from build123d import *

# Parameters (mm, degrees)
F1_DEPTH     = 19.05
F2_R         = 15.059033574
F3_DEPTH     = 3.81
F6_DEPTH     = 25.4
F8_DEPTH     = 98.4172728563
F4_R         = 4.2206847971
F9_DEPTH     = 25.4
F10_SIZE     = 3.80999
F11_R        = 12.7
F12_R        = 12.7
F13_R        = 7.62
F14_R        = 5.08
F15_R        = 7.62
F16_R        = 7.62
F17_R        = 5.08
F18_R        = 7.62
F19_R        = 5.08
F20_T1_DEPTH = 19.05
F21_R        = 2.54
F22_R        = 15.24


# Not quite as in the source:
# - a fillet or chamfer that OpenCascade refuses, or shapes differently, is made with other operations: its cross-section is extruded or revolved along the edge and cut away or added
# - a fillet or chamfer is up to 0.001 mm smaller than in the source, because OpenCascade refuses the exact size


with BuildPart() as f1:
    # F0 (on Top) → F1 (new body)
    with BuildSketch(Plane.XY):
        Polygon((57.15, 90.8419879414), (0, 90.8419879414), (-57.15, 90.8419879414), (-47.625, -86.9580120586), (0, -86.9580120586), (47.625, -86.9580120586), align=None)
        with BuildLine():
            Line((-39.8510134111, -64.9218410254), (-19.0060128585, -64.9218410254))
            ThreePointArc((-19.0060128585, -64.9218410254), (-15.7100075961, -71.1253052436), (-10.4695623741, -75.8033767343))
            Line((-10.4695623741, -75.8033767343), (-10.4695623741, -78.8165818754))
            Line((-10.4695623741, -78.8165818754), (-40.5953745281, -78.8165818754))
            Line((-40.5953745281, -78.8165818754), (-39.8510134111, -64.9218410254))
        make_face(mode=Mode.SUBTRACT)
        with BuildLine():
            Line((-42.0940332115, -10.5141438544), (-10.4695623741, -10.5141438544))
            Line((-10.4695623741, -10.5141438544), (-10.4695623741, -41.7985618114))
            ThreePointArc((-10.4695623741, -41.7985618114), (-15.6132317705, -46.3542592872), (-18.9080441845, -52.3838467943))
            Line((-18.9080441845, -52.3838467943), (-39.8510134111, -52.3838467943))
            Line((-39.8510134111, -52.3838467943), (-42.0940332115, -10.5141438544))
        make_face(mode=Mode.SUBTRACT)
        with BuildLine():
            Line((19.0060128585, -64.9218410254), (39.8510134111, -64.9218410254))
            Line((39.8510134111, -64.9218410254), (40.5953745281, -78.8165818754))
            Line((40.5953745281, -78.8165818754), (10.4695623741, -78.8165818754))
            Line((10.4695623741, -78.8165818754), (10.4695623741, -75.8033767343))
            ThreePointArc((10.4695623741, -75.8033767343), (15.7100075961, -71.1253052436), (19.0060128585, -64.9218410254))
        make_face(mode=Mode.SUBTRACT)
        with BuildLine():
            Line((10.4695623741, -10.5141438544), (42.0940332115, -10.5141438544))
            Line((42.0940332115, -10.5141438544), (39.8510134111, -52.3838467943))
            Line((39.8510134111, -52.3838467943), (18.9080441845, -52.3838467943))
            ThreePointArc((18.9080441845, -52.3838467943), (15.6132317705, -46.3542592872), (10.4695623741, -41.7985618114))
            Line((10.4695623741, -41.7985618114), (10.4695623741, -10.5141438544))
        make_face(mode=Mode.SUBTRACT)
        Polygon((-10.4695623741, 71.0973963141), (-10.4695623741, 4.7880196944), (-42.0940332115, 4.7880196944), (-45.4945191741, 71.0973963141), align=None, mode=Mode.SUBTRACT)
        Polygon((10.4695623741, 4.7880196944), (10.4695623741, 71.0973963141), (45.4945191741, 71.0973963141), (42.0940332115, 4.7880196944), align=None, mode=Mode.SUBTRACT)
    extrude(amount=F1_DEPTH)

    # F2 (on face) → F3 (join)
    with BuildSketch(Plane.XY.offset(19.05)):
        with Locations((0, -58.8009692729)):
            Circle(F2_R)
    extrude(amount=F3_DEPTH)

    # F5 (on face) → F6 (join)
    with BuildSketch(Plane.XY.offset(19.05)):
        Polygon((15.6109640375, 85.8776420355), (0, 85.8776420355), (-15.6109640375, 85.8776420355), (-15.6109640375, 76.2544423342), (0, 76.2544423342), (15.6109640375, 76.2544423342), align=None)
        Polygon((-15.6109640375, -7.5742849149), (0, -7.5742849149), (15.6109640375, -7.5742849149), (15.6109640375, 2.0489108283), (0, 2.0489108283), (-15.6109640375, 2.0489108283), align=None)
    extrude(amount=F6_DEPTH)

    # F7 (on face) → F8 (cut, through all)
    with BuildSketch(Plane.XZ.offset(7.5742849149)):
        Polygon((3.81, 35.5143319389), (0, 35.5143319389), (-3.81, 35.5143319389), (-3.81, 27.8943319389), (0, 27.8943319389), (3.81, 27.8943319389), align=None)
    extrude(amount=-F8_DEPTH, mode=Mode.SUBTRACT)

    # F4 (on face) → F9 (join)
    with BuildSketch(Plane.XY.offset(22.86)):
        with Locations((0, -58.8009692729)):
            Circle(F4_R)
    extrude(amount=F9_DEPTH)

    # F10 (size 3.81 in the source; OpenCascade refuses exactly that, so slightly less here)
    f10_edges = [f1.edges().sort_by_distance(p)[0] for p in [
        (-15.059034, -58.800969, 22.86),
    ]]
    chamfer(f10_edges, length=F10_SIZE)

    # F11
    f11_edges = [f1.edges().sort_by_distance(p)[0] for p in [
        (15.610964, -2.762687, 44.45),
        (-15.610964, -2.762687, 44.45),
    ]]
    fillet(f11_edges, radius=F11_R)

    # F12
    f12_edges = [f1.edges().sort_by_distance(p)[0] for p in [
        (15.610964, 81.066042, 44.45),
        (-15.610964, 81.066042, 44.45),
    ]]
    fillet(f12_edges, radius=F12_R)

    # F13
    f13_edges = [f1.edges().sort_by_distance(p)[0] for p in [
        (-45.494519, 71.097396, 9.525),
    ]]
    fillet(f13_edges, radius=F13_R)

    # F14
    f14_edges = [f1.edges().sort_by_distance(p)[0] for p in [
        (-42.094033, -10.514144, 9.525),
    ]]
    fillet(f14_edges, radius=F14_R)

    # F15
    f15_edges = [f1.edges().sort_by_distance(p)[0] for p in [
        (-10.469562, 71.097396, 9.525),
        (45.494519, 71.097396, 9.525),
    ]]
    fillet(f15_edges, radius=F15_R)

    # F16
    f16_edges = [f1.edges().sort_by_distance(p)[0] for p in [
        (-42.094033, 4.78802, 9.525),
        (10.469562, 4.78802, 9.525),
    ]]
    fillet(f16_edges, radius=F16_R)

    # F17
    f17_edges = [f1.edges().sort_by_distance(p)[0] for p in [
        (-10.469562, 4.78802, 9.525),
        (42.094033, 4.78802, 9.525),
    ]]
    fillet(f17_edges, radius=F17_R)

    # F18
    f18_edges = [f1.edges().sort_by_distance(p)[0] for p in [
        (10.469562, 71.097396, 9.525),
    ]]
    fillet(f18_edges, radius=F18_R)

    # F19
    f19_edges = [f1.edges().sort_by_distance(p)[0] for p in [
        (-10.469562, -10.514144, 9.525),
        (42.094033, -10.514144, 9.525),
        (10.469562, -10.514144, 9.525),
        (-39.851013, -52.383847, 9.525),
        (39.851013, -52.383847, 9.525),
    ]]
    fillet(f19_edges, radius=F19_R)

    # F20: fillet of radius 5.08 on 6 edges, made by hand

    # F20_s2 → F20_t1 (join)
    with BuildSketch(Plane.XY):
        with BuildLine():
            ThreePointArc((40.3086734646, -73.4648286909), (38.9228773885, -77.2312845683), (35.2359473527, -78.8165818754))
            Line((35.2359473527, -78.8165818754), (40.5953745281, -78.8165818754))
            Line((40.5953745281, -78.8165818754), (40.3086734646, -73.4648286909))
        make_face()
        with BuildLine():
            ThreePointArc((-15.1101182687, -78.8165818754), (-12.3436148694, -77.9971990774), (-10.4695623741, -75.8033767343))
            Line((-10.4695623741, -75.8033767343), (-10.4695623741, -78.8165818754))
            Line((-10.4695623741, -78.8165818754), (-15.1101182687, -78.8165818754))
        make_face()
        with BuildLine():
            ThreePointArc((-40.3086734646, -73.4648286909), (-38.9228773885, -77.2312845683), (-35.2359473527, -78.8165818754))
            Line((-35.2359473527, -78.8165818754), (-40.5953745281, -78.8165818754))
            Line((-40.5953745281, -78.8165818754), (-40.3086734646, -73.4648286909))
        make_face()
        with BuildLine():
            ThreePointArc((10.4695623741, -75.8033767343), (12.3436148694, -77.9971990774), (15.1101182687, -78.8165818754))
            Line((15.1101182687, -78.8165818754), (10.4695623741, -78.8165818754))
            Line((10.4695623741, -78.8165818754), (10.4695623741, -75.8033767343))
        make_face()
        with BuildLine():
            ThreePointArc((35.03587195, -64.9218410254), (38.5305746428, -66.3149109896), (40.1085980619, -69.7300878408))
            Line((40.1085980619, -69.7300878408), (39.8510134111, -64.9218410254))
            Line((39.8510134111, -64.9218410254), (35.03587195, -64.9218410254))
        make_face()
        with BuildLine():
            ThreePointArc((-35.03587195, -64.9218410254), (-38.5305746428, -66.3149109896), (-40.1085980619, -69.7300878408))
            Line((-40.1085980619, -69.7300878408), (-39.8510134111, -64.9218410254))
            Line((-39.8510134111, -64.9218410254), (-35.03587195, -64.9218410254))
        make_face()
    extrude(amount=F20_T1_DEPTH)

    # F21
    f21_edges = [f1.edges().sort_by_distance(p)[0] for p in [
        (10.469562, -75.803377, 9.525),
        (-10.469562, -75.803377, 9.525),
    ]]
    fillet(f21_edges, radius=F21_R)

    # F22
    f22_edges = [f1.edges().sort_by_distance(p)[0] for p in [
        (-47.625, -86.958012, 9.525),
        (-57.15, 90.841988, 9.525),
        (57.15, 90.841988, 9.525),
        (47.625, -86.958012, 9.525),
    ]]
    fillet(f22_edges, radius=F22_R)


solid = f1.part
The model under review builds one solid part; all positions refer to its coordinate system, in mm. A direction names the side the tool comes from. Give positions to 0.01 mm unless a question says otherwise; leave off trailing zeros. Write each loop counter-clockwise with the first axis right and the second up, starting at its lowest first coordinate (ties: lowest second). Pieces come first, ordered by that corner, then holes.
1. Wall thickness on L1, parallel to Y at x = 28.5, z = 15; L2, parallel to Y at x = -38.5, z = 10; L3, parallel to Z at x = -1.5, y = 0.5: over which ranges is each line inside the solid? List them lowest first.
2. For P1, Ø3, axis at x = 12.5, z = 41, coming from the +Y side; P2, Ø4, axis at x = 28, y = 69.5, coming from the +Z side; P3, Ø4, axis at y = 58.5, z = 6.5, coming from the -X side; P4, Ø8, axis at x = 35.5, z = 6.5, coming from the -Y side, all flat-tipped, find the tip position at first contact; note any pin that passes through.
3. Draft analysis for pull direction Z (two halves, no side actions). For faces 1 (the flat face through (5, -59, 22.86)), 2 (the flat face through (0, -3, 35.514)), 3 (the flat face through (-28, 71.097, 9)), state which applies: +Z half, -Z half, draft (parallel to the pull), parting line (faces both ways), or undercut.
4. Add section C-C, the plane x = 28.5. Write out the cut boundary in (y, z), plus the area to 3 significant figures.
5. Add section A-A, the plane x = 0. Count the separate pieces of the cut face and the enclosed holes in it, plus the area to 3 significant figures.
6. Add section B-B, the plane y = 60. Write out the cut boundary in (x, z).
7. Tool access review of faces 4 (the cylindrical face through (16.48, -70.075, 9.392)), 5 (the flat face through (0, -3, 27.894)), 6 (the flat face through (1, 90.842, 9)): name each direction out of +Z, -Z, +X, -X, +Y, -Y from which nothing blocks a thin tool from reaching the whole face with its end or side.
Worked answers:
1. L1: y = -86.96 to -78.82, -64.92 to -52.38, -10.51 to 4.79, 71.1 to 90.84
1. L2: y = -86 to -77.63, -66.29 to -51.02, -10.83 to 5.72, 71.03 to 90.84
1. L3: z = 0 to 27.89, 35.51 to 44.45
2. P1: stops at y = 85.88
2. P2: stops at z = 19.05
2. P3: stops at x = -55.52
2. P4: stops at y = -86.96
3. face 1: +Z half
3. face 2: undercut
3. face 3: draft
4. outline: (-86.96, 0) - (-78.82, 0) - (-78.82, 19.05) - (-86.96, 19.05) - close; (-64.92, 0) - (-52.38, 0) - (-52.38, 19.05) - (-64.92, 19.05) - close; (-10.51, 0) - (4.79, 0) - (4.79, 19.05) - (-10.51, 19.05) - close; (71.1, 0) - (90.84, 0) - (90.84, 19.05) - (71.1, 19.05) - close
4. area: 1,060 mm2
5. separate pieces: 3
5. enclosed holes: 0
5. area: 4,040 mm2
6. outline: (-55.5, 0) - (-44.93, 0) - (-44.93, 19.05) - (-55.5, 19.05) - close; (-10.47, 0) - (10.47, 0) - (10.47, 19.05) - (-10.47, 19.05) - close; (44.93, 0) - (55.5, 0) - (55.5, 19.05) - (44.93, 19.05) - close
7. face 4: +Z, -Z
7. face 5: +Y
7. face 6: +Z, -Z, +X, -X, +Y
